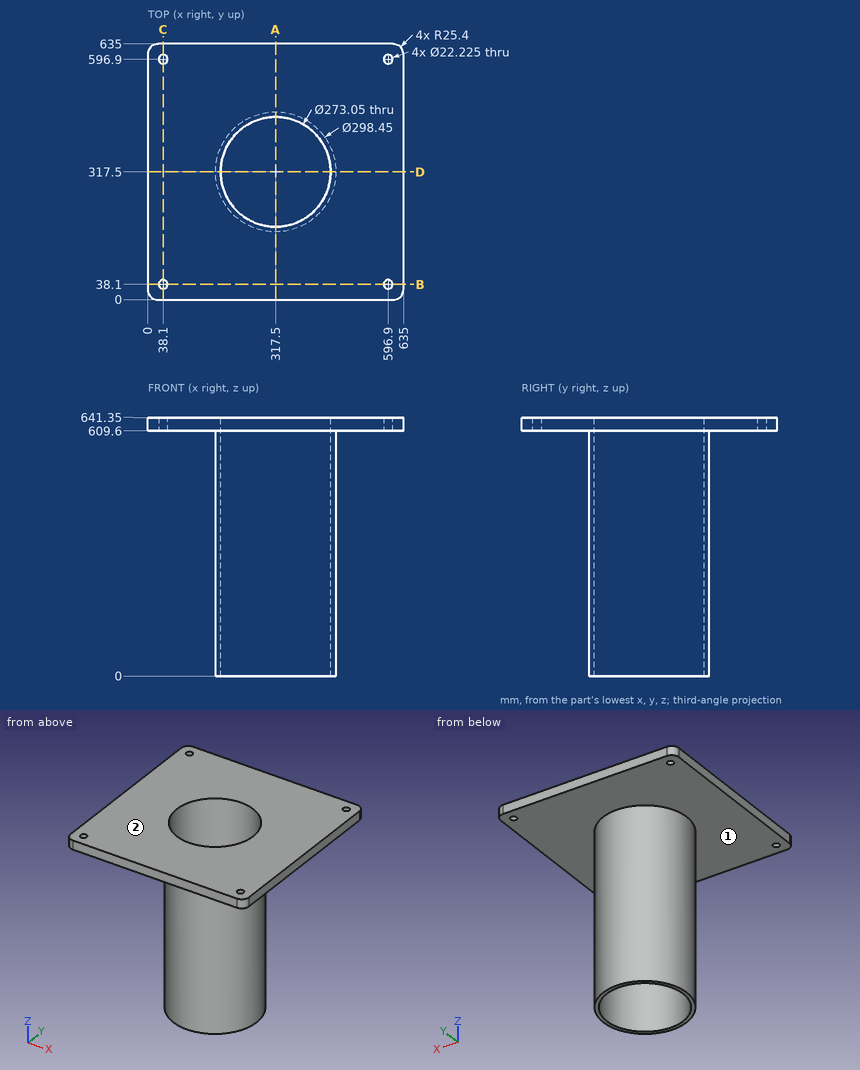
Source: three-view drawing plus pictorial views. Frame: mm from the lowest corner of the part. A direction names the side the tool comes from. Coordinates: 2 decimals unless noted, no trailing zeros. Order: outer loops, then holes, each group sorted by start corner. A loop starts at its lowest first (then second) coordinate and runs counter-clockwise, first axis right, second up. Notation, with made-up numbers: (39.25, 86) -> (57.25, 86) arc R30 cw to (57.25, 114) -> close; hole circle Ø3 at (-29, 51.5). An arc over 180 degrees is marked (long way). Write item = value, one per line.
(1) Line query: line 1 (Y direction, x = 38.1, z = 633); line 2 (Z direction, x = 532.5, y = 227.5); line 3 (Y direction, x = 200, z = 252.5). Output: solid intervals per line, ascending.
Solved:
line_1 = 0 to 26.99, 49.21 to 585.79, 608.01 to 635
line_2 = 609.6 to 641.35
line_3 = 225.51 to 247.98, 387.02 to 409.49
(2) Pin query (flat end, axial travel): pin 1 Ø1.5 at (x, y) = (465, 372) entering from -Z; pin 2 Ø2 at (y, z) = (264.5, 574) entering from +X; pin 3 Ø1.5 at (y, z) = (267.5, 150) entering from +X. Return the tip coordinate at first contact, or that it passes through.
Solved:
pin_1 = 609.6
pin_2 = 457.37
pin_3 = 458.36
(3) Cut plane B-B on y = 38.1. Return loops of the section in (x, z), plus the area to 4 significant figures.
Solved:
outline = (0, 609.6) -> (26.99, 609.6) -> (26.99, 641.35) -> (0, 641.35) -> close; (49.21, 609.6) -> (585.79, 609.6) -> (585.79, 641.35) -> (49.21, 641.35) -> close; (608.01, 609.6) -> (635, 609.6) -> (635, 641.35) -> (608.01, 641.35) -> close
area = 18,750 mm²
(4) Cut plane A-A on x = 317.5. Return loops of the section in (y, z) (3 decimals).
Solved:
outline = (0, 609.6) -> (168.275, 609.6) -> (168.275, 0) -> (180.975, 0) -> (180.975, 641.35) -> (0, 641.35) -> close; (454.025, 0) -> (466.725, 0) -> (466.725, 609.6) -> (635, 609.6) -> (635, 641.35) -> (454.025, 641.35) -> close
(5) Access query for the marked faces 1 and 2. Directions: +Z, -Z, +X, -X, +Y, -Y. A direction counts if a zero-diameter tool reaches every point of the face in a straight line with its end or side. Return the directions, or none.
Solved:
face_1 = -Z
face_2 = +Z, +X, -X, +Y, -Y
